The figure shows three views and two pictorial views of one solid part (mm, origin at its lowest corner). Answer the questions. Coordinates: 2 decimals unless noted, no trailing zeros. Write each loop counter-clockwise with the first axis right and the second up, starting at its lowest first coordinate (ties: lowest second). Pieces come first, ordered by that corner, then holes. Notation, with made-up numbers: M 8,-5.5 L 28,-5.5 A20 cw 28,3.5 Z; hole C 8,34 d2. An arc over 180 degrees is marked long. Use a Markdown table: item, result. Add a question column.
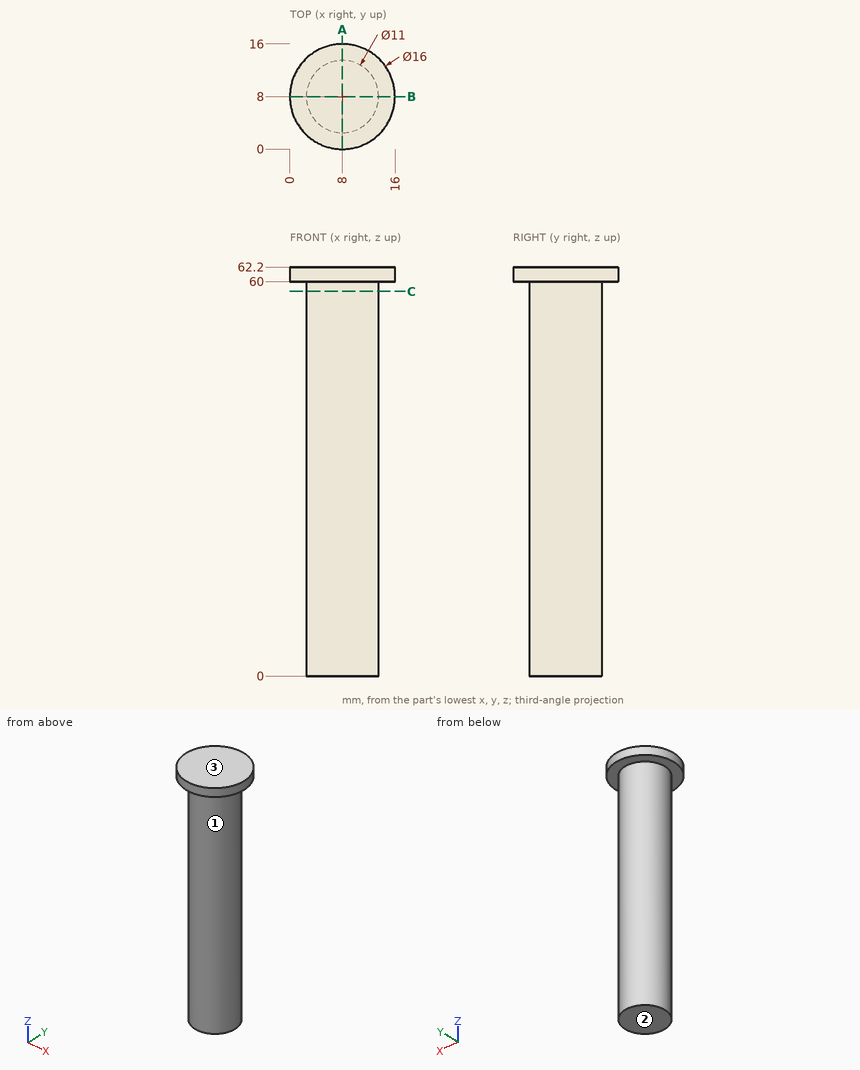
Item 1: Determine the mould class of the marked faces 1, 2 and 3 for opening direction Z: pulls with the +Z half, pulls with the -Z half, needs draft (parallel to the pull), parting line crosses it, or undercut.
Item 2: Find section A-A on x = 8. Give the vertices of the cut face in (y, z), then the cut area to 3 significant figures.
Item 3: Consider probe 1 along Z at (x, y) = (9, 14.5); probe 2 along Y at (x, z) = (10.5, 10); probe 3 along Y at (x, z) = (4.5, 34.5). Determine where each line is inside the solid, lowest interval first.
Item 4: Each of these flat-tipped pins is pushed along its axis until it touches: pin 1 (8 mm diameter, centred on y = 6, z = 48, fed in from -X); pin 2 (8 mm diameter, centred on x = 9.5, z = 53, fed in from +Y); pin 3 (3 mm diameter, centred on y = 5, z = 13.5, fed in from -X). Where does it stop, or does it pass through?
Item 5: Find section C-C on z = 58.5. Give the vertices of the cut face in (x, y), then the cut area to 3 significant figures.
Geometry says:
| question | item | result |
|---|---|---|
| 1 | face 1 | needs draft |
| 1 | face 2 | pulls with the -Z half |
| 1 | face 3 | pulls with the +Z half |
| 2 | outline | M 0,60 L 2.5,60 L 2.5,0 L 13.5,0 L 13.5,60 L 16,60 L 16,62.2 L 0,62.2 Z |
| 2 | area | 695 mm2 |
| 3 | probe 1 | z = 60 to 62.2 |
| 3 | probe 2 | y = 3.1 to 12.9 |
| 3 | probe 3 | y = 3.76 to 12.24 |
| 4 | pin 1 | stops at x = 2.5 |
| 4 | pin 2 | stops at y = 13.5 |
| 4 | pin 3 | stops at x = 2.71 |
| 5 | outline | C 8,8 d11 |
| 5 | area | 95.0 mm2 |
